```python
from build123d import *

# Parameters (mm, degrees)
SKETCH_1_R           = 1.1
SKETCH_1_R_2         = 4
EXTRUDE_1_DEPTH      = 2.5
SKETCH_2_W           = 14.4
SKETCH_2_H           = 0.5
CUT_EXTRUDE_1_DEPTH  = 37.005863078
SKETCH_3_W           = 13
SKETCH_3_H           = 1.3
CUT_EXTRUDE_2_DEPTH  = 4.5
SKETCH_4_W           = 13
SKETCH_4_H           = 1.3
CUT_EXTRUDE_3_DEPTH  = 4.5
SKETCH_5_W           = 11.5
SKETCH_5_H           = 17.3
CUT_EXTRUDE_11_DEPTH = 0.5
SKETCH_6_W           = 6
SKETCH_6_H           = 10
CUT_EXTRUDE_12_DEPTH = 0.5
FILLET_1_R           = 0.5
FILLET_2_R           = 1


with BuildPart() as part:
    # 草图1 → 凸台-拉伸1 (new body)
    with BuildSketch(Plane(origin=(0, 0, 0), x_dir=(1, 0, 0), z_dir=(0, 1, 0))):
        with BuildLine():
            Line((-12, 24.224), (-12, -10.776))
            ThreePointArc((-12, -10.776), (-11.267766953, -12.543766953), (-9.5, -13.276))
            Line((-9.5, -13.276), (9.5, -13.276))
            ThreePointArc((9.5, -13.276), (11.267766953, -12.543766953), (12, -10.776))
            Line((12, -10.776), (12, 24.224))
            ThreePointArc((12, 24.224), (11.267766953, 25.991766953), (9.5, 26.724))
            Line((9.5, 26.724), (-9.5, 26.724))
            ThreePointArc((-9.5, 26.724), (-11.267766953, 25.991766953), (-12, 24.224))
        make_face()
        with Locations(Location((-9.714, -10.986, 0), (0, 0, 270))):
            Circle(SKETCH_1_R, mode=Mode.SUBTRACT)
        with Locations(Location((0, 0.32, 0), (0, 0, 270))):
            Circle(SKETCH_1_R_2, mode=Mode.SUBTRACT)
        with Locations(Location((9.714, -10.986, 0), (0, 0, 270))):
            Circle(SKETCH_1_R, mode=Mode.SUBTRACT)
        with Locations(Location((9.714, 10.986, 0), (0, 0, 270))):
            Circle(SKETCH_1_R, mode=Mode.SUBTRACT)
        with Locations(Location((-9.714, 10.986, 0), (0, 0, 270))):
            Circle(SKETCH_1_R, mode=Mode.SUBTRACT)
    extrude(amount=-EXTRUDE_1_DEPTH)

    # 草图2 → 切除-拉伸1 (cut, through all)
    with BuildSketch(Plane(origin=(12, 0, 0), x_dir=(0, 0, -1), z_dir=(1, 0, 0))):
        with Locations((0.924, -2.25)):
            Rectangle(SKETCH_2_W, SKETCH_2_H)
    extrude(amount=-CUT_EXTRUDE_1_DEPTH, mode=Mode.SUBTRACT)

    # 草图3 → 切除-拉伸2 (cut)
    with BuildSketch(Plane(origin=(12, 0, 0), x_dir=(0, 0, -1), z_dir=(1, 0, 0))):
        with Locations((1.624, -1.85)):
            Rectangle(SKETCH_3_W, SKETCH_3_H)
    extrude(amount=-CUT_EXTRUDE_2_DEPTH, mode=Mode.SUBTRACT)

    # 草图4 → 切除-拉伸3 (cut)
    with BuildSketch(Plane.ZY.offset(12)):
        with Locations((-1.624, -1.85)):
            Rectangle(SKETCH_4_W, SKETCH_4_H)
    extrude(amount=-CUT_EXTRUDE_3_DEPTH, mode=Mode.SUBTRACT)

    # 草图5 → 切除-拉伸11 (cut)
    with BuildSketch(Plane.XZ.offset(2.5)):
        with Locations((1.75, -16.774)):
            Rectangle(SKETCH_5_W, SKETCH_5_H)
    extrude(amount=-CUT_EXTRUDE_11_DEPTH, mode=Mode.SUBTRACT)

    # 草图6 → 切除-拉伸12 (cut)
    with BuildSketch(Plane.XZ.offset(2)):
        with Locations((-1, -13.124)):
            Rectangle(SKETCH_6_W, SKETCH_6_H)
    extrude(amount=-CUT_EXTRUDE_12_DEPTH, mode=Mode.SUBTRACT)

    # 圆角1
    # the kernel refuses this fillet: 0.5 mm, written as the material it takes off along each edge
    with BuildSketch(Plane(origin=(-9.5, 0, 13.276), x_dir=(0, 0, -1), z_dir=(1, 0, 0))) as fillet_1_piece_1:
        with BuildLine():
            CenterArc((FILLET_1_R, -FILLET_1_R), FILLET_1_R, 90, 90)
            Line((0, -FILLET_1_R), (-FILLET_1_R * 0.02, -FILLET_1_R))
            Line((-FILLET_1_R * 0.02, -FILLET_1_R), (-FILLET_1_R * 0.02, FILLET_1_R * 0.02))
            Line((-FILLET_1_R * 0.02, FILLET_1_R * 0.02), (FILLET_1_R, FILLET_1_R * 0.02))
            Line((FILLET_1_R, FILLET_1_R * 0.02), (FILLET_1_R, 0))
        make_face()
    extrude(amount=19, mode=Mode.SUBTRACT)
    with BuildSketch(Plane(origin=(-9.5, 0, 10.776), x_dir=(-1, 0, 0), z_dir=(0, 0, -1))) as fillet_1_piece_2:
        with BuildLine():
            CenterArc((2.5 - FILLET_1_R, -FILLET_1_R), FILLET_1_R, 0, 90)
            Line((2.5, -FILLET_1_R), (2.5 + FILLET_1_R * 0.02, -FILLET_1_R))
            Line((2.5 + FILLET_1_R * 0.02, -FILLET_1_R), (2.5 + FILLET_1_R * 0.02, FILLET_1_R * 0.02))
            Line((2.5 + FILLET_1_R * 0.02, FILLET_1_R * 0.02), (2.5 - FILLET_1_R, FILLET_1_R * 0.02))
            Line((2.5 - FILLET_1_R, FILLET_1_R * 0.02), (2.5 - FILLET_1_R, 0))
        make_face()
    revolve(axis=Axis((-9.5, 0, 10.776), (0, 1, 0)), revolution_arc=90, mode=Mode.SUBTRACT)
    with BuildSketch(Plane(origin=(-12, 0, -27.224), x_dir=(0, -1, 0), z_dir=(0, 0, 1))) as fillet_1_piece_3:
        with BuildLine():
            CenterArc((FILLET_1_R, FILLET_1_R), FILLET_1_R, 180, 90)
            Line((0, FILLET_1_R), (-FILLET_1_R * 0.02, FILLET_1_R))
            Line((-FILLET_1_R * 0.02, FILLET_1_R), (-FILLET_1_R * 0.02, -FILLET_1_R * 0.02))
            Line((-FILLET_1_R * 0.02, -FILLET_1_R * 0.02), (FILLET_1_R, -FILLET_1_R * 0.02))
            Line((FILLET_1_R, -FILLET_1_R * 0.02), (FILLET_1_R, 0))
        make_face()
    extrude(amount=38, mode=Mode.SUBTRACT)
    with BuildSketch(Plane(origin=(12, 0, 10.776), x_dir=(-1, 0, 0), z_dir=(0, 0, -1))) as fillet_1_piece_4:
        with BuildLine():
            CenterArc((FILLET_1_R, -FILLET_1_R), FILLET_1_R, 90, 90)
            Line((0, -FILLET_1_R), (-FILLET_1_R * 0.02, -FILLET_1_R))
            Line((-FILLET_1_R * 0.02, -FILLET_1_R), (-FILLET_1_R * 0.02, FILLET_1_R * 0.02))
            Line((-FILLET_1_R * 0.02, FILLET_1_R * 0.02), (FILLET_1_R, FILLET_1_R * 0.02))
            Line((FILLET_1_R, FILLET_1_R * 0.02), (FILLET_1_R, 0))
        make_face()
    extrude(amount=38, mode=Mode.SUBTRACT)
    with BuildSketch(Plane(origin=(9.5, 0, 10.776), x_dir=(0, 0, 1), z_dir=(-1, 0, 0))) as fillet_1_piece_5:
        with BuildLine():
            CenterArc((2.5 - FILLET_1_R, -FILLET_1_R), FILLET_1_R, 0, 90)
            Line((2.5, -FILLET_1_R), (2.5 + FILLET_1_R * 0.02, -FILLET_1_R))
            Line((2.5 + FILLET_1_R * 0.02, -FILLET_1_R), (2.5 + FILLET_1_R * 0.02, FILLET_1_R * 0.02))
            Line((2.5 + FILLET_1_R * 0.02, FILLET_1_R * 0.02), (2.5 - FILLET_1_R, FILLET_1_R * 0.02))
            Line((2.5 - FILLET_1_R, FILLET_1_R * 0.02), (2.5 - FILLET_1_R, 0))
        make_face()
    revolve(axis=Axis((9.5, 0, 10.776), (0, 1, 0)), revolution_arc=90, mode=Mode.SUBTRACT)

    # 圆角2
    fillet_2_edges = [part.edges().sort_by_distance(p)[0] for p in [
        (0, 0, -4.32),
    ]]
    fillet(fillet_2_edges, radius=FILLET_2_R)


solid = part.part
```
Geometry: final body of the model. Coordinates: model frame, mm. A direction names the side the tool comes from. Round coordinates to 2 decimals unless told otherwise and drop trailing zeros. Order: outer loops, then holes, each group sorted by start corner. A loop starts at its lowest first (then second) coordinate and runs counter-clockwise, first axis right, second up. Notation, with made-up numbers: M 7.25,-39.75 L 63.25,-39.75 A24 cw 63.25,-19.75 Z; hole C -5.5,-36 d5. An arc over 180 degrees is marked long. Use one line per item in the form item = value. Start each with the question number.
Q1. Pin query (flat end, axial travel): pin 1 Ø5 at (x, z) = (-9, -2.5) entering from -Y; pin 2 Ø0.9 at (y, z) = (-1.5, 0) entering from -X. Return the tip coordinate at first contact, or that it passes through.
Q2. Cut plane C-C (x = -9). Return loops of the section in (y, z), and give its area (3 significant figures).
Q3. Mould query, pull axis X, two halves, no side actions, for faces 4 (the face through (0, -1, 13.276)), 5 (the face through (-8.623, -1.232, 10.843)), 6 (the face through (12, -1, -6)), 7 (the face through (-11.25, -1.23, -26.01)). Classes: +X half, -X half, draft (parallel to the pull), parting line (faces both ways), or undercut.
Q4. Access query for faces 1 (the face through (10, -1.2, -2)), 2 (the face through (-4, -2, -15)), 3 (the face through (-9, -2, -8.124)). Directions: +Z, -Z, +X, -X, +Y, -Y. A direction counts if a zero-diameter tool reaches every point of the face in a straight line with its end or side. Return the directions, or none.
Q5. Cut plane D-D (z = -16). Return loops of the section in (x, y).
Q6. Cut plane B-B (x = 0). Return loops of the section in (y, z).
Q7. Material intervals for line 1 (X direction, y = -2.3, z = -11); line 2 (X direction, y = -0.5, z = -11.5); line 3 (Z direction, x = 5, y = -2.15), sorted ascending. Write a range as [from, to].
Q8. Cut plane A-A (z = -0.32). Return loops of the section in (x, y).
Geometry results:
q1.pin_1 = -2
q1.pin_2 = -12
q2.outline = M -2.5,-26.72 L 0,-26.72 L 0,-11.82 L -2.5,-11.82 Z; M -2.5,-10.15 L 0,-10.15 L 0,10.15 L -2.5,10.15 L -2.5,6.28 L -2,6.28 L -2,4.88 L -1.2,4.88 L -1.2,-8.12 L -2.5,-8.12 Z; M -2.5,11.82 L 0,11.82 L 0,12.78 A0.5 ccw -0.5,13.28 L -2.5,13.28 Z
q2.area = 74.0 mm^2
q3.face_4 = draft
q3.face_5 = undercut
q3.face_6 = +X half
q3.face_7 = -X half
q4.face_1 = +X, -Y
q4.face_2 = -Y
q4.face_3 = -X, -Y
q5.outline = M -12,-2.5 L -4,-2.5 L -4,-1.5 L 2,-1.5 L 2,-2 L 7.5,-2 L 7.5,-2.5 L 12,-2.5 L 12,-0.5 A0.5 ccw 11.5,0 L -11.5,0 A0.5 ccw -12,-0.5 Z
q6.outline = M -2.5,-26.72 L 0,-26.72 L 0,-5.32 A1 ccw -1,-4.32 L -2,-4.32 L -2,-8.12 L -1.5,-8.12 L -1.5,-18.12 L -2,-18.12 L -2,-25.42 L -2.5,-25.42 Z; M -2.5,6.28 L -2,6.28 L -2,3.68 L -1,3.68 A1 ccw 0,4.68 L 0,12.78 A0.5 ccw -0.5,13.28 L -2.5,13.28 Z
q7.line_1 = [-12, -10.81], [-8.61, -4], [7.5, 8.61], [10.81, 12]
q7.line_2 = [-12, -10.69], [-8.74, 8.74], [10.69, 12]
q7.line_3 = [-26.72, -25.42], [6.28, 13.28]
q8.outline = M -12,-1.2 L -7.5,-1.2 L -7.5,-2 L -4,-2 L -4,-1 A1 ccw -5,0 L -11.5,0 A0.5 ccw -12,-0.5 Z; M 4,-2 L 7.5,-2 L 7.5,-1.2 L 12,-1.2 L 12,-0.5 A0.5 ccw 11.5,0 L 5,0 A1 ccw 4,-1 Z
